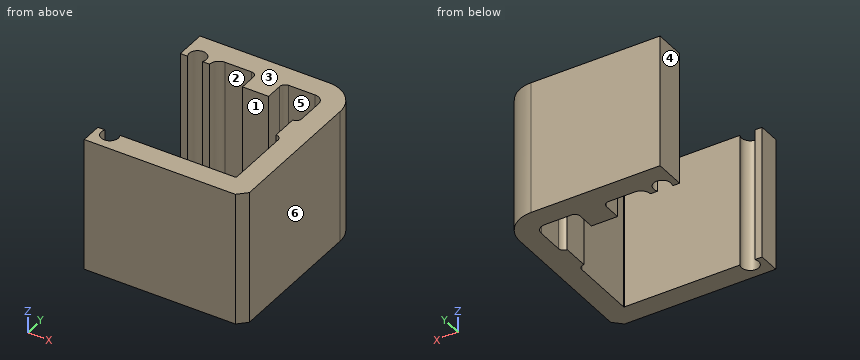
Autodesk Inventor part; units mm, degrees
ref_plane "YZ Plane" through (0, 0, 0) normal (1, 0, 0) x (0, 1, 0)
ref_plane "XZ Plane" through (0, 0, 0) normal (0, 1, 0) x (-1, 0, 0)
ref_plane "XY Plane" through (0, 0, 0) normal (0, 0, 1) x (1, 0, 0)
ref_plane "Work Plane2" through (0, 0, -200) normal (0, 0, 1) x (1, 0, 0)
ref_plane "Work Plane1" through (0, 0, 0) normal (0, 0, 1) x (1, 0, 0)
sketch "Sketch1" plane through (0, 0, -200) normal (0, 0, 1) x (1, 0, 0)
  arc A0 (6.1983, 20.8783) -> (6.1983, 23.0183) centre (6.1983, 21.9483) ccw construction
  line L0 (12.2867, 14.8983) -> (8.7499, 14.8983) construction
  arc A1 (14.8383, 23.0183) -> (14.8383, 20.8783) centre (14.8383, 21.9483) ccw construction
  arc A2 (23.0183, 21.0366) -> (21.0366, 23.0183) centre (21.0366, 21.0366) ccw construction
  line L1 (21.0366, 23.0183) -> (14.8383, 23.0183) construction
  arc A3 (20.8783, 14.8383) -> (23.0183, 14.8383) centre (21.9483, 14.8383) ccw construction
  line L2 (23.0183, 14.8383) -> (23.0183, 21.0366) construction
  line L3 (14.8983, 8.7499) -> (14.8983, 12.2867) construction
  line L4 (-1.9817, 21.0366) -> (-1.9817, 0) construction
  arc A4 (-1.9817, 0) -> (0, -1.9817) centre (0, 0) ccw construction
  line L5 (0, -1.9817) -> (6.1983, -1.9817) construction
  line L6 (14.8383, -1.9817) -> (21.0366, -1.9817) construction
  arc A5 (21.0366, -1.9817) -> (23.0183, 0) centre (21.0366, 0) ccw construction
  line L7 (23.0183, 0) -> (23.0183, 6.1983) construction
  arc A6 (23.0183, 6.1983) -> (20.8783, 6.1983) centre (21.9483, 6.1983) ccw construction
  line L8 (20.8783, 6.1983) -> (20.8783, 4.0901) construction
  arc A7 (19.1681, 3.3817) -> (20.8783, 4.0901) centre (19.8765, 4.0901) ccw construction
  line L9 (19.1681, 3.3817) -> (15.675, 6.8748) construction
  arc A8 (14.8983, 8.7499) -> (15.675, 6.8748) centre (17.55, 8.7499) ccw construction
  line L10 (15.675, 14.1617) -> (19.1681, 17.6549) construction
  arc A9 (15.675, 14.1617) -> (14.8983, 12.2867) centre (17.55, 12.2867) ccw construction
  line L11 (20.8783, 16.9465) -> (20.8783, 14.8383) construction
  arc A10 (20.8783, 16.9465) -> (19.1681, 17.6549) centre (19.8765, 16.9465) ccw construction
  line L12 (17.6549, 19.1681) -> (14.1617, 15.675) construction
  arc A11 (17.6549, 19.1681) -> (16.9465, 20.8783) centre (16.9465, 19.8765) ccw construction
  line L13 (14.8383, 20.8783) -> (16.9465, 20.8783) construction
  arc A12 (12.2867, 14.8983) -> (14.1617, 15.675) centre (12.2867, 17.55) ccw construction
  arc A13 (6.8748, 15.675) -> (8.7499, 14.8983) centre (8.7499, 17.55) ccw construction
  line L14 (6.8748, 15.675) -> (3.3817, 19.1681) construction
  arc A14 (4.0901, 20.8783) -> (3.3817, 19.1681) centre (4.0901, 19.8765) ccw construction
  line L15 (4.0901, 20.8783) -> (6.1983, 20.8783) construction
  line L16 (6.1983, 23.0183) -> (0, 23.0183) construction
  arc A15 (0, 23.0183) -> (-1.9817, 21.0366) centre (0, 21.0366) ccw construction
  line L17 (7.4683, 21.9483) -> (7.4683, 17.8983)
  line L18 (7.4683, 17.8983) -> (13.5683, 17.8983)
  line L19 (13.5683, 17.8983) -> (13.5683, 21.9483)
  arc A16 (7.4683, 21.9483) -> (6.1983, 23.2183) centre (6.1983, 21.9483) ccw
  arc A17 (14.8383, 23.2183) -> (13.5683, 21.9483) centre (14.8383, 21.9483) ccw
  line L20 (6.1983, 23.2183) -> (0, 23.2183)
  line L21 (0, 23.2183) -> (0, 28.2183)
  line L22 (0, 28.2183) -> (21.0366, 28.2183)
  arc A18 (23.2183, 21.0366) -> (21.0366, 23.2183) centre (21.0366, 21.0366) ccw
  line L23 (23.2183, 21.0366) -> (23.2183, 14.8383)
  arc A19 (21.9483, 13.5683) -> (23.2183, 14.8383) centre (21.9483, 14.8383) ccw
  arc A20 (28.2183, 21.0366) -> (21.0366, 28.2183) centre (21.0366, 21.0366) ccw
  line L24 (28.2183, 21.0366) -> (28.2183, 0)
  line L25 (21.9483, 13.5683) -> (21.9483, 7.4683)
  arc A21 (23.2183, 6.1983) -> (21.9483, 7.4683) centre (21.9483, 6.1983) ccw
  line L26 (23.2183, 6.1983) -> (23.2183, -8.9287)
  line L27 (23.0183, -9.1287) -> (-9, -9.1287)
  line L28 (-9, -9.1287) -> (-9, -14.1287)
  line L29 (-9, -14.1287) -> (26.2183, -14.1287)
  line L30 (28.2183, -12.1287) -> (28.2183, 0)
  arc A22 (23.0183, -9.1287) -> (23.2183, -8.9287) centre (23.0183, -8.9287) ccw
  line L31 (14.8383, 23.2183) -> (21.0366, 23.2183)
  line L32 (0, 28.2183) -> (-9, 28.2183)
  arc A23 (0, 23.2183) -> (-2.1817, 21.0366) centre (0, 21.0366) ccw
  line L33 (-2.1817, 21.0366) -> (-9, 21.0366)
  line L34 (-9, 21.0366) -> (-9, 28.2183)
  circle A24 centre (-5.5909, 22.0366) radius 2
  line L35 (-5.5909, 21.0366) -> (-5.5909, 28.2183) construction
  line L36 (-5.5909, 21.0366) -> (-5.5909, -14.1287) construction
  circle A25 centre (-5.5909, -10.1287) radius 2
  line L37 (26.2183, -14.1287) -> (28.2183, -12.1287)
  point P0 (0, 0)
  point P1 (7.2683, 21.9483)
  point P2 (10.5183, 14.8983)
  point P3 (10.5183, 17.8983)
  point P4 (13.7683, 21.9483)
  point P5 (23.0183, -8.9287)
  point P6 (-1.9817, -8.9287)
  point P7 (28.2183, -14.1287)
  point P8 (17.4722, 23.2183)
  point P9 (-9, 24.6274)
  point P10 (-3.8588, -9.1287)
  point P11 (-7.3229, -9.1287)
  point P12 (-7.3229, 21.0366)
  point P13 (-3.8588, 21.0366)
  dimension "d1" = 0.2
  dimension "d2" = 3
  dimension "d3" = 0.2
  dimension "d4" = 0.2
  dimension "d5" = 0.2
  dimension "d6" = 5
  dimension "d7" = 5
  dimension "d8" = 5
  dimension "d9" = 0.2
  dimension "d13" = 9
  dimension "d14" = 4
  dimension "d15" = 1
  dimension "d16" = 4
  dimension "d17" = 1
  dimension "d18" = 135
  dimension "d19" = 2
extrude "Extrusion1" add sketch "Sketch1" along normal blind 31 contours A16 L20 L21 L22 A20 L24 L30 L37 L29 L28 L27 A25 A22 L26 A21 L25 A19 L23 A18 L31 A17 L19 L18 L17 | A23 L33 A24 L34 L32 L21
properties part number "HangerNinety"
Verification items for the finished model (mm, model axes). Face numbers are marked on the shaded views. A direction names the side the tool comes from. Round coordinates to 2 decimals unless told otherwise and drop trailing zeros. Loops run counter-clockwise (first coordinate to the right, second up) from the corner with the lowest first, then second, coordinate; pieces in that order, holes last. Notation, with made-up numbers: (-29, 15) - (-9, 15) arc R20 cw to (-9, 22) - close; hole circle Ø8 at (39, 12.25). An arc over 180 degrees is marked (long way). Use one line per item in the form item = value.
1. Access from +Z, -Z, +X, -X, +Y, -Y to the whole of each face (thin tool, end or side, straight path). Record for the marked faces 1, 2 and 3.
A:
face_1 = +Z, -Z, -X
face_2 = +Z, -Z
face_3 = +Z, +X, -X, +Y, -Y
2. Gauge pin test, flat ends, axial feed: pin 1 Ø10 at (y, z) = (11.5, -172.5) entering from -X; pin 2 Ø3 at (y, z) = (19.5, -180) entering from -X; pin 3 Ø1 at (y, z) = (-3.5, -176) entering from -X. Record the tip position at first contact, or that the pin passes through.
A:
pin_1 = 21.95
pin_2 = 7.47
pin_3 = 23.22
3. Section check C-C on y = -10. Record the cut outline in (x, z).
A:
outline = (-9, -200) - (-7.59, -200) - (-7.59, -169) - (-9, -169) - close; (-3.6, -200) - (28.22, -200) - (28.22, -169) - (-3.6, -169) - close
4. Section check B-B on z = -183. Record the cut outline in (x, y).
A:
outline = (-9, -14.13) - (26.22, -14.13) - (28.22, -12.13) - (28.22, 21.04) arc R7.18 ccw to (21.04, 28.22) - (-9, 28.22) - (-9, 21.04) - (-7.32, 21.04) arc R2 cw (long way) to (-3.86, 21.04) - (-2.18, 21.04) arc R2.18 cw to (0, 23.22) - (6.2, 23.22) arc R1.27 cw to (7.47, 21.95) - (7.47, 17.9) - (13.57, 17.9) - (13.57, 21.95) arc R1.27 cw to (14.84, 23.22) - (21.04, 23.22) arc R2.18 cw to (23.22, 21.04) - (23.22, 14.84) arc R1.27 cw to (21.95, 13.57) - (21.95, 7.47) arc R1.27 cw to (23.22, 6.2) - (23.22, -8.93) arc R0.2 cw to (23.02, -9.13) - (-3.86, -9.13) arc R2 cw (long way) to (-7.32, -9.13) - (-9, -9.13) - close
5. Section check D-D on x = 22.5. Record the cut outline in (y, z).
A:
outline = (-14.13, -200) - (-9.13, -200) - (-9.13, -169) - (-14.13, -169) - close; (7.34, -200) - (13.69, -200) - (13.69, -169) - (7.34, -169) - close; (22.65, -200) - (28.07, -200) - (28.07, -169) - (22.65, -169) - close
6. Draft check along X on the marked faces 4, 5 and 6. Enter one of: pulls with the +X half, pulls with the -X half, needs draft (parallel to the pull), parting line crosses it, or undercut.
A:
face_4 = pulls with the -X half
face_5 = undercut
face_6 = pulls with the +X half
7. Section check A-A on x = 5. Record the cut outline in (y, z).
A:
outline = (-14.13, -200) - (-9.13, -200) - (-9.13, -169) - (-14.13, -169) - close; (23.22, -200) - (28.22, -200) - (28.22, -169) - (23.22, -169) - close
8. Scan lines: probe 1 along Y at (x, z) = (8, -185.5); probe 2 along Y at (x, z) = (-3, -188); probe 3 along X at (y, z) = (23, -194). Record each from-to range of solid material in increasing order.
A:
probe_1 = -14.13 to -9.13, 17.9 to 28.22
probe_2 = -14.13 to -9.13, 21.04 to 28.22
probe_3 = -9 to -7.34, -3.84 to -0.95, 6.91 to 14.13, 21.99 to 27.94
